from build123d import *

# Parameters (mm, degrees)
SKETCH1_W           = 76.2
SKETCH1_H           = 76.2
SKETCH1_R           = 5
SKETCH1_R_2         = 3.175
BOSS_EXTRUDE1_DEPTH = 3


with BuildPart() as part:
    # Sketch1 → Boss-Extrude1 (new body)
    # profile 1 of 5: a face of its own
    with BuildSketch(Plane(origin=(0, 0, 0), x_dir=(1, 0, 0), z_dir=(0, 1, 0))):
        Rectangle(SKETCH1_W, SKETCH1_H)
        with Locations((31.730846191, 31.730846191)):
            Circle(SKETCH1_R, mode=Mode.SUBTRACT)
        with Locations((-31.730846191, 31.730846191)):
            Circle(SKETCH1_R, mode=Mode.SUBTRACT)
        with Locations((-31.730846191, -31.730846191)):
            Circle(SKETCH1_R, mode=Mode.SUBTRACT)
        with Locations((31.730846191, -31.730846191)):
            Circle(SKETCH1_R, mode=Mode.SUBTRACT)
        with Locations(Location((0, 0, 0), (0, 0, 270))):
            Circle(SKETCH1_R_2, mode=Mode.SUBTRACT)
    # profile 2 of 5: a face of its own
    with BuildSketch(Plane(origin=(0, 0, 0), x_dir=(1, 0, 0), z_dir=(0, 1, 0))):
        with Locations((-31.730846191, 31.730846191)):
            Circle(SKETCH1_R)
    # profile 3 of 5: a face of its own
    with BuildSketch(Plane(origin=(0, 0, 0), x_dir=(1, 0, 0), z_dir=(0, 1, 0))):
        with Locations((31.730846191, 31.730846191)):
            Circle(SKETCH1_R)
    # profile 4 of 5: a face of its own
    with BuildSketch(Plane(origin=(0, 0, 0), x_dir=(1, 0, 0), z_dir=(0, 1, 0))):
        with Locations((31.730846191, -31.730846191)):
            Circle(SKETCH1_R)
    # profile 5 of 5: a face of its own
    with BuildSketch(Plane(origin=(0, 0, 0), x_dir=(1, 0, 0), z_dir=(0, 1, 0))):
        with Locations((-31.730846191, -31.730846191)):
            Circle(SKETCH1_R)
    extrude(amount=BOSS_EXTRUDE1_DEPTH)


solid = part.part
The listing builds one solid part. Answer for the finished solid, in the listing's coordinates (mm). Give positions to 0.01 mm unless a question says otherwise; leave off trailing zeros. Order: outer loops, then holes, each group sorted by start corner. A loop starts at its lowest first (then second) coordinate and runs counter-clockwise, first axis right, second up. Notation, with made-up numbers: (7.25, -19) - (26.25, -19) arc R20 cw to (26.25, -15) - close; hole circle Ø11 at (55, 63.25). An arc over 180 degrees is marked (long way). Use one line per item in the form item = value.
1) The mould has two halves that part along Z. Classify faces 1 (the flat face through (-1, 1, 38.1)), 2 (the flat face through (-38.1, 1, 1)), 3 (the cylindrical face through (-1.93, 1.48, -2.52)): released by +Z, released by -Z, zero draft, split by the parting line, or undercut.
Verdict:
face_1 = released by +Z
face_2 = zero draft
face_3 = undercut
2) Find section B-B on z = 0. Determine the outline of the cut face in (x, y) (3 decimals), and give its area (3 significant figures).
Verdict:
outline = (-38.1, 0) - (-3.175, 0) - (-3.175, 3) - (-38.1, 3) - close; (3.175, 0) - (38.1, 0) - (38.1, 3) - (3.175, 3) - close
area = 210 mm^2
3) Find section A-A on x = 0. Determine the outline of the cut face in (y, z) (3 decimals), and give its area (3 significant figures).
Verdict:
outline = (0, -38.1) - (3, -38.1) - (3, -3.175) - (0, -3.175) - close; (0, 3.175) - (3, 3.175) - (3, 38.1) - (0, 38.1) - close
area = 210 mm^2
4) Consider probe 1 along X at (y, z) = (1.25, 0) (3 decimals); probe 2 along Z at (x, y) = (-1, 2.25). Determine where each line is inside the solid, lowest interval first. Write a range as [from, to].
Verdict:
probe_1 = [-38.1, -3.175], [3.175, 38.1]
probe_2 = [-38.1, -3.01], [3.01, 38.1]
